Check sheet for the modelled part. Datum: model origin and axes. Units: mm. A direction names the side the tool comes from. Give positions to 0.01 mm unless a question says otherwise; leave off trailing zeros. Write each loop counter-clockwise with the first axis right and the second up, starting at its lowest first coordinate (ties: lowest second). Pieces come first, ordered by that corner, then holes. Notation, with made-up numbers: M 64,50 L 80,50 A23 cw 80,85 Z; hole C 73.5,-30.5 d4. An arc over 180 degrees is marked long. One line per item, written item: value. Start each with the question number.
from build123d import *

# Parameters (mm, degrees)
F1_DEPTH = 7.62
F2_R     = 1.5875
F3_R     = 1.5875
F4_DEPTH = 25.4
F2_R_2   = 2.921
F3_R_2   = 2.921
F5_DEPTH = 2.794
F6_ANGLE = -90


with BuildPart() as f1:
    # F0 (on Top) → F1 (new body)
    with BuildSketch(Plane.XY):
        with BuildLine():
            Line((11.43, 1.27), (12.6363404513, 1.27))
            ThreePointArc((12.6363404513, 1.27), (12.2207385876, 3.4559439194), (11.43, 5.5358016583))
            Line((11.43, 5.5358016583), (11.43, 1.27))
        make_face()
        with BuildLine():
            ThreePointArc((11.43, 5.5358016583), (12.2207385876, 3.4559439194), (12.6363404513, 1.27))
            Line((12.6363404513, 1.27), (19.05, 1.27))
            Line((19.05, 1.27), (19.05, 7.62))
            Line((19.05, 7.62), (11.43, 7.62))
            Line((11.43, 7.62), (11.43, 5.5358016583))
        make_face()
        with BuildLine():
            Line((11.43, 1.27), (11.43, 5.5358016583))
            ThreePointArc((11.43, 5.5358016583), (10.8451830635, 6.6084797282), (10.16, 7.62))
            Line((10.16, 7.62), (5.0545361805, 7.62))
            ThreePointArc((5.0545361805, 7.62), (7.7364740689, 4.8743927807), (9.0553760827, 1.27))
            Line((9.0553760827, 1.27), (11.43, 1.27))
        make_face()
        with BuildLine():
            ThreePointArc((10.16, 7.62), (10.8451830635, 6.6084797282), (11.43, 5.5358016583))
            Line((11.43, 5.5358016583), (11.43, 7.62))
            Line((11.43, 7.62), (10.16, 7.62))
        make_face()
        with BuildLine():
            Line((5.0545361805, 7.62), (10.16, 7.62))
            ThreePointArc((10.16, 7.62), (0, 12.7), (-10.16, 7.62))
            Line((-10.16, 7.62), (-5.0545361805, 7.62))
            ThreePointArc((-5.0545361805, 7.62), (0, 9.144), (5.0545361805, 7.62))
        make_face()
        with BuildLine():
            Line((-5.0545361805, 7.62), (-10.16, 7.62))
            ThreePointArc((-10.16, 7.62), (-10.8451830635, 6.6084797282), (-11.43, 5.5358016583))
            Line((-11.43, 5.5358016583), (-11.43, 1.27))
            Line((-11.43, 1.27), (-9.0553760827, 1.27))
            ThreePointArc((-9.0553760827, 1.27), (-7.7364740689, 4.8743927807), (-5.0545361805, 7.62))
        make_face()
        with BuildLine():
            ThreePointArc((-11.43, 5.5358016583), (-10.8451830635, 6.6084797282), (-10.16, 7.62))
            Line((-10.16, 7.62), (-11.43, 7.62))
            Line((-11.43, 7.62), (-11.43, 5.5358016583))
        make_face()
        with BuildLine():
            Line((-11.43, 1.27), (-11.43, 5.5358016583))
            ThreePointArc((-11.43, 5.5358016583), (-12.2207385876, 3.4559439194), (-12.6363404513, 1.27))
            Line((-12.6363404513, 1.27), (-11.43, 1.27))
        make_face()
        with BuildLine():
            ThreePointArc((-12.6363404513, 1.27), (-12.2207385876, 3.4559439194), (-11.43, 5.5358016583))
            Line((-11.43, 5.5358016583), (-11.43, 7.62))
            Line((-11.43, 7.62), (-19.05, 7.62))
            Line((-19.05, 7.62), (-19.05, 1.27))
            Line((-19.05, 1.27), (-12.6363404513, 1.27))
        make_face()
    extrude(amount=F1_DEPTH)

    # F2 (on face) + F3 (on face) → F4 (cut)
    with BuildSketch(Plane(origin=(0, 7.62, 0), x_dir=(-1, 0, 0), z_dir=(0, 1, 0))):
        with Locations((-15.24, 3.81)):
            Circle(F2_R)
    with BuildSketch(Plane(origin=(0, 7.62, 0), x_dir=(-1, 0, 0), z_dir=(0, 1, 0))):
        with Locations((15.24, 3.81)):
            Circle(F3_R)
    extrude(amount=-F4_DEPTH, mode=Mode.SUBTRACT)

    # F2 (on face) + F3 (on face) → F5 (cut)
    with BuildSketch(Plane(origin=(0, 7.62, 0), x_dir=(-1, 0, 0), z_dir=(0, 1, 0))):
        with Locations((-15.24, 3.81)):
            Circle(F2_R_2)
        with Locations((-15.24, 3.81)):
            Circle(F2_R, mode=Mode.SUBTRACT)
    with BuildSketch(Plane(origin=(0, 7.62, 0), x_dir=(-1, 0, 0), z_dir=(0, 1, 0))):
        with Locations((15.24, 3.81)):
            Circle(F3_R_2)
        with Locations((15.24, 3.81)):
            Circle(F3_R, mode=Mode.SUBTRACT)
    extrude(amount=-F5_DEPTH, mode=Mode.SUBTRACT)


with BuildPart() as f1_1:
    # F6: moved
    add(f1.part.rotate(Axis((19.05, 1.27, 3.81), (0, 0, -1)), F6_ANGLE))


solid = f1_1.part
1) Gauge pin test, flat ends, axial feed: pin 1 (2.5 mm diameter, centred on y = -33.02, z = 3.81, fed in from -X); pin 2 (1 mm diameter, centred on y = -20.5, z = 5.5, fed in from +X); pin 3 (3 mm diameter, centred on y = -34, z = 3, fed in from -X); pin 4 (4 mm diameter, centred on y = -4.5, z = 2.5, fed in from -X). Record the tip position at first contact, or that the pin passes through.
2) Cross-section at C-C (x = 17.25). Record the boundary of the cut face in (y, z) (1 decimal), plus the area to 3 significant figures.
3) Cross-section at A-A (z = 3.81). Record the boundary of the cut face in (x, y).
4) Cross-section at D-D (x = 12.25). Record the boundary of the cut face in (y, z), plus the area to 3 significant figures.
5) Cross-section at B-B (y = -2.54). Record the boundary of the cut face in (x, z), plus the area to 3 significant figures.
6) Draft check along Y on faces 1 (the flat face through (16, 1.27, 4)), 2 (the cylindrical face through (14.077, -35.806, 4.687)), 3 (the flat face through (19.05, -31, 4)), 4 (the flat face through (15.494, -3.8, 2.6)). Enter one of: released by +Y, released by -Y, zero draft, split by the parting line, or undercut.
7) Material ranges on L1, parallel to Z at x = 14.7, y = -2.54; L2, parallel to Z at x = 16.25, y = -33.02; L3, parallel to Y at x = 16, z = 5, recorded low to high. Write a range as from..to.
8) Tool access check on faces 5 (the flat face through (16, -36.83, 4)), 6 (the flat face through (12.7, -5.1, 2.1)), 7 (the cylindrical face through (17.247, -34.534, 4.287)), 8 (the flat face through (15.494, -34.3, 2.6)), 9 (the flat face through (12.7, -30, 2)). Record the directions out of +Z, -Z, +X, -X, +Y, -Y that give a thin tool (end or side, any length) a straight path to the whole face; none if there is none.
Data:
1. pin 1: passes through
1. pin 2: stops at x = 11.76
1. pin 3: stops at x = 15.49
1. pin 4: stops at x = 12.7
2. outline: M -36.8,0 L -26.4,0 L -26.4,7.6 L -36.8,7.6 Z; M -9.2,0 L 1.3,0 L 1.3,7.6 L -9.2,7.6 Z; hole C -33,3.8 d3.2; hole C -2.5,3.8 d3.2
2. area: 143 mm2
3. outline: M 12.7,-36.83 L 19.05,-36.83 L 19.05,-34.61 L 15.49,-34.61 L 15.49,-35.94 L 12.7,-35.94 Z; M 12.7,-30.1 L 15.49,-30.1 L 15.49,-31.43 L 19.05,-31.43 L 19.05,-26.84 A9.14 cw 19.05,-8.72 L 19.05,-4.13 L 15.49,-4.13 L 15.49,-5.46 L 12.7,-5.46 L 12.7,-7.62 A12.7 ccw 12.7,-27.94 Z; M 12.7,0.38 L 15.49,0.38 L 15.49,-0.95 L 19.05,-0.95 L 19.05,1.27 L 12.7,1.27 Z
4. outline: M -27.59,0 L -22.08,0 L -22.08,7.62 L -27.59,7.62 Z; M -13.48,0 L -7.97,0 L -7.97,7.62 L -13.48,7.62 Z
4. area: 83.9 mm2
5. outline: M 12.7,0 L 19.05,0 L 19.05,2.22 L 15.49,2.22 L 15.49,0.89 L 12.7,0.89 Z; M 12.7,6.73 L 15.49,6.73 L 15.49,5.4 L 19.05,5.4 L 19.05,7.62 L 12.7,7.62 Z
5. area: 20.8 mm2
6. face 1: released by +Y
6. face 2: undercut
6. face 3: zero draft
6. face 4: undercut
7. L1: z = 0..0.89, 6.73..7.62
7. L2: z = 0..2.22, 5.4..7.62
7. L3: y = -36.83..-34.07, -31.97..-25.84, -9.72..-3.59, -1.49..1.27
8. face 5: +Z, -Z, +X, -X, -Y
8. face 6: +Z, -Z, -X, +Y
8. face 7: +X, -X
8. face 8: -X
8. face 9: +Z, -Z, -X, -Y
